Design review of the part built by this model. Coordinates are the model's own, in mm. A direction names the side the tool comes from. Round coordinates to 2 decimals unless told otherwise and drop trailing zeros. Order: outer loops, then holes, each group sorted by start corner. A loop starts at its lowest first (then second) coordinate and runs counter-clockwise, first axis right, second up. Notation, with made-up numbers: (43.25, 19.25) - (98.25, 19.25) arc R16 ccw to (98.25, 23.25) - close; hole circle Ø1 at (29.5, -37). An arc over 180 degrees is marked (long way). Write item = value, one per line.
from build123d import *

# Parameters (mm, degrees)
SKETCH_1_W           = 86
SKETCH_1_H           = 25
EXTRUDE_1_DEPTH      = 7
SKETCH_2_W           = 15
SKETCH_2_H           = 17
CUT_EXTRUDE_1_DEPTH  = 90.833178726
SKETCH_3_W           = 55
SKETCH_3_H           = 13
CUT_EXTRUDE_2_DEPTH  = 5.2
SKETCH_4_W           = 55
SKETCH_4_H           = 7.5
CUT_EXTRUDE_3_DEPTH  = 2
CHAMFER_1_SIZE       = 1
SKETCH_5_R           = 1.8
CUT_EXTRUDE_4_DEPTH  = 90.699498326
SKETCH_6_R           = 1.4
CUT_EXTRUDE_5_DEPTH  = 90.699498326
CUT_EXTRUDE_6_DEPTH  = 90.710868907
SKETCH_8_W           = 7
SKETCH_8_H           = 6
EXTRUDE_2_DEPTH      = 7.55
SKETCH_9_R           = 2
CUT_EXTRUDE_7_DEPTH  = 91.734241056
SKETCH_10_W          = 14.55
SKETCH_10_H          = 6
SKETCH_10_R          = 1.75
EXTRUDE_3_DEPTH      = 7
EXTRUDE_START        = -7
SKETCH_12_W          = 14.55
SKETCH_12_H          = 6
SKETCH_12_R          = 1.75
EXTRUDE_5_DEPTH      = 7
SKETCH_13_W          = 7
SKETCH_13_H          = 6
CUT_EXTRUDE_8_DEPTH  = 3
SKETCH_14_W          = 7
SKETCH_14_H          = 6
CUT_EXTRUDE_9_DEPTH  = 3
CUT_EXTRUDE_10_DEPTH = 15


with BuildPart() as part:
    # 草图1 → 凸台-拉伸1 (new body)
    with BuildSketch(Plane.XY):
        with Locations((43, 12.5)):
            Rectangle(SKETCH_1_W, SKETCH_1_H)
    extrude(amount=EXTRUDE_1_DEPTH)

    # 草图2 → 切除-拉伸1 (cut, through all)
    with BuildSketch(Plane.XY.offset(7)):
        with Locations((16.5, 10.5)):
            Rectangle(SKETCH_2_W, SKETCH_2_H)
    extrude(amount=-CUT_EXTRUDE_1_DEPTH, mode=Mode.SUBTRACT)

    # 草图3 → 切除-拉伸2 (cut)
    with BuildSketch(Plane.XY.offset(7)):
        with Locations((51.5, 8.5)):
            Rectangle(SKETCH_3_W, SKETCH_3_H)
    extrude(amount=-CUT_EXTRUDE_2_DEPTH, mode=Mode.SUBTRACT)

    # 草图4 → 切除-拉伸3 (cut)
    with BuildSketch(Plane.XY.offset(7)):
        with Locations((51.5, 18.75)):
            Rectangle(SKETCH_4_W, SKETCH_4_H)
    extrude(amount=-CUT_EXTRUDE_3_DEPTH, mode=Mode.SUBTRACT)

    # 倒角1
    chamfer_1_edges = [part.edges().sort_by_distance(p)[0] for p in [
        (51.5, 15, 5),
    ]]
    chamfer(chamfer_1_edges, length=CHAMFER_1_SIZE)

    # 草图5 → 切除-拉伸4 (cut, through all)
    with BuildSketch(Plane.XY.offset(5)):
        with Locations((30, 18)):
            Circle(SKETCH_5_R)
        with Locations((39.5, 18)):
            Circle(SKETCH_5_R)
        with Locations((70.5, 18)):
            Circle(SKETCH_5_R)
    extrude(amount=-CUT_EXTRUDE_4_DEPTH, mode=Mode.SUBTRACT)

    # 草图6 → 切除-拉伸5 (cut, through all)
    with BuildSketch(Plane.XY.offset(5)):
        with Locations((35, 18)):
            Circle(SKETCH_6_R)
        with Locations((65.5, 18)):
            Circle(SKETCH_6_R)
    extrude(amount=-CUT_EXTRUDE_5_DEPTH, mode=Mode.SUBTRACT)

    # 草图7 → 切除-拉伸6 (cut, through all)
    with BuildSketch(Plane.XY.offset(1.8)):
        with BuildLine():
            Line((29, 11.5), (46, 11.5))
            ThreePointArc((46, 11.5), (49, 8.5), (46, 5.5))
            Line((46, 5.5), (29, 5.5))
            ThreePointArc((29, 5.5), (26, 8.5), (29, 11.5))
        make_face()
        with BuildLine():
            Line((54, 11.5), (71, 11.5))
            ThreePointArc((71, 11.5), (74, 8.5), (71, 5.5))
            Line((71, 5.5), (54, 5.5))
            ThreePointArc((54, 5.5), (51, 8.5), (54, 11.5))
        make_face()
    extrude(amount=-CUT_EXTRUDE_6_DEPTH, mode=Mode.SUBTRACT)

    # 草图8 → 凸台-拉伸2 (add)
    with BuildSketch(Plane.XY.offset(7)):
        with Locations((3.5, 22)):
            Rectangle(SKETCH_8_W, SKETCH_8_H)
        with Locations((82.5, 3)):
            Rectangle(SKETCH_8_W, SKETCH_8_H)
        with Locations((3.5, 3)):
            Rectangle(SKETCH_8_W, SKETCH_8_H)
        with Locations((82.5, 22)):
            Rectangle(SKETCH_8_W, SKETCH_8_H)
    extrude(amount=EXTRUDE_2_DEPTH)

    # 草图9 → 切除-拉伸7 (cut, through all)
    with BuildSketch(Plane.XY.offset(14.55)):
        with Locations((3.5, 22)):
            Circle(SKETCH_9_R)
        with Locations((82.5, 3)):
            Circle(SKETCH_9_R)
        with Locations((82.5, 22)):
            Circle(SKETCH_9_R)
        with Locations((3.5, 3)):
            Circle(SKETCH_9_R)
    extrude(amount=-CUT_EXTRUDE_7_DEPTH, mode=Mode.SUBTRACT)

    # 草图10 → 凸台-拉伸3 (add)
    # profile 1 of 2: a face of its own
    with BuildSketch(Plane.ZY):
        with Locations((7.275, 28)):
            Rectangle(SKETCH_10_W, SKETCH_10_H)
        with Locations((11.05, 28)):
            Circle(SKETCH_10_R, mode=Mode.SUBTRACT)
    # profile 2 of 2: a face of its own
    with BuildSketch(Plane.ZY):
        with Locations((7.275, -3)):
            Rectangle(SKETCH_10_W, SKETCH_10_H)
        with Locations((11.05, -3)):
            Circle(SKETCH_10_R, mode=Mode.SUBTRACT)
    extrude(amount=-EXTRUDE_3_DEPTH)

    # 草图12 → 凸台-拉伸5 (add)
    # profile 1 of 2: a face of its own
    with BuildSketch(Plane(origin=(86, 0, 0), x_dir=(0, 0, -1), z_dir=(1, 0, 0)).offset(EXTRUDE_START)):
        with Locations((-7.275, 28)):
            Rectangle(SKETCH_12_W, SKETCH_12_H)
        with Locations(Location((-11.05, 28, 0), (0, 0, 180))):
            Circle(SKETCH_12_R, mode=Mode.SUBTRACT)
    # profile 2 of 2: a face of its own
    with BuildSketch(Plane(origin=(86, 0, 0), x_dir=(0, 0, -1), z_dir=(1, 0, 0)).offset(EXTRUDE_START)):
        with Locations((-7.275, -3)):
            Rectangle(SKETCH_12_W, SKETCH_12_H)
        with Locations(Location((-11.05, -3, 0), (0, 0, 180))):
            Circle(SKETCH_12_R, mode=Mode.SUBTRACT)
    extrude(amount=EXTRUDE_5_DEPTH)

    # 草图13 → 切除-拉伸8 (cut)
    with BuildSketch(Plane.ZY):
        with Locations((3.5, 12.5)):
            Rectangle(SKETCH_13_W, SKETCH_13_H)
    extrude(amount=-CUT_EXTRUDE_8_DEPTH, mode=Mode.SUBTRACT)

    # 草图14 → 切除-拉伸9 (cut)
    with BuildSketch(Plane(origin=(86, 0, 0), x_dir=(0, 0, -1), z_dir=(1, 0, 0))):
        with Locations((-3.5, 12.5)):
            Rectangle(SKETCH_14_W, SKETCH_14_H)
    extrude(amount=-CUT_EXTRUDE_9_DEPTH, mode=Mode.SUBTRACT)

    # 草图20 → 切除-拉伸10 (cut)
    with BuildSketch(Plane.ZY.offset(-24)):
        Polygon((0, 19), (7, 19), (7, 22), (3, 25), (0, 25), align=None)
    extrude(amount=CUT_EXTRUDE_10_DEPTH, mode=Mode.SUBTRACT)


solid = part.part
Item 1: For line 1 along Y through (x, z) = (3.5, 5.5); line 2 along Y through (x, z) = (30, 3); line 3 along X through (y, z) = (27, 2.5), list the stretches that pass through material, from the lowest coordinate up. Write a range as [from, to].
Data:
line_1 = [-6, 1], [5, 20], [24, 31]
line_2 = [0, 2], [15, 16.2], [19.8, 25]
line_3 = [0, 7], [79, 86]
Item 2: Take a section at A-A, the plane x = 35. State the section outline as (y, z) points, and give its area (3 significant figures).
Data:
outline = (0, 0) - (5.5, 0) - (5.5, 1.8) - (2, 1.8) - (2, 7) - (0, 7) - close; (11.5, 0) - (16.6, 0) - (16.6, 5) - (16, 5) - (15, 4) - (15, 1.8) - (11.5, 1.8) - close; (19.4, 0) - (25, 0) - (25, 7) - (22.5, 7) - (22.5, 5) - (19.4, 5) - close
area = 67.1 mm2
Item 3: For faces 4 (the face through (51, 15, 3)), 5 (the face through (3, 19, 11)), 6 (the face through (42, 0, 3)), 7 (the face through (51, 8.4, 0.9)), list the 3-axis set-ups (+Z, -Z, +X, -X, +Y, -Y) from which the entire face can be reached by the end or side of a thin tool; tool diameter is ignored.
Data:
face_4 = +Z
face_5 = +Z, +X, -X
face_6 = +Z, -Z, -Y
face_7 = +Z, -Z
Item 4: The part is to be moulded in two halves that separate along X. For faces 1 (the face through (3.45, 29.18, 9.76)), 2 (the face through (86, 2, 7)), 3 (the face through (24, 16, 2)), say which applies: +X half, -X half, draft (parallel to the pull), parting line (faces both ways), or undercut.
Data:
face_1 = draft
face_2 = +X half
face_3 = undercut
Item 5: Take a section at D-D, the plane z = 11.5. Count the separate pieces of the cut face and the enclosed holes in it, and give its area (3 significant figures).
Data:
separate_pieces = 8
enclosed_holes = 4
area = 191 mm2
Item 6: Take a section at B-B, the plane y = 8. State the section outline as (x, z) points, and give its area (3 significant figures).
Data:
outline = (0, 0) - (9, 0) - (9, 7) - (0, 7) - close; (24, 0) - (26.04, 0) - (26.04, 1.8) - (24, 1.8) - close; (48.96, 0) - (51.04, 0) - (51.04, 1.8) - (48.96, 1.8) - close; (73.96, 0) - (86, 0) - (86, 7) - (79, 7) - (79, 1.8) - (73.96, 1.8) - close
area = 129 mm2
Item 7: Take a section at C-C, the plane x = 52.5. State the section outline as (y, z) points, and give its area (3 significant figures).
Data:
outline = (0, 0) - (5.9, 0) - (5.9, 1.8) - (2, 1.8) - (2, 7) - (0, 7) - close; (11.1, 0) - (25, 0) - (25, 7) - (22.5, 7) - (22.5, 5) - (16, 5) - (15, 4) - (15, 1.8) - (11.1, 1.8) - close
area = 82.5 mm2
Item 8: Insertion check: P1, Ø7.5, axis at x = 60, z = 2, coming from the +Y side; P2, Ø5, axis at y = 8.5, z = 8, coming from the -X side; P3, Ø2, axis at x = 53, z = 4.5, coming from the -Y side; P4, Ø1.9, axis at y = 11.5, z = 2.5, coming from the -X side. Each pin has a flat end and moves straight along its axis. Give the tip position at first contact, or say it passes through.
Data:
P1 = 25
P2 = 0
P3 = 0
P4 = 3
